Design review of the part built by this model. Coordinates are the model's own, in mm. Coordinates: 2 decimals unless noted, no trailing zeros. Order: outer loops, then holes, each group sorted by start corner. A loop starts at its lowest first (then second) coordinate and runs counter-clockwise, first axis right, second up. Notation, with made-up numbers: M 38.5,-2.75 L 77.5,-2.75 A19 cw 77.5,9.25 Z; hole C 0.25,-33.5 d11. An arc over 180 degrees is marked long. Answer in a Markdown table with one row per item.
from build123d import *

# Parameters (mm, degrees)
SKETCH1_R           = 3.05
SKETCH1_R_2         = 1.27
BOSS_EXTRUDE1_DEPTH = 5
FILLET1_R           = 3
SKETCH2_R           = 1.3
CUT_EXTRUDE1_DEPTH  = 339.464178311


with BuildPart() as part:
    # Sketch1 → Boss-Extrude1 (new body)
    with BuildSketch(Plane.XY):
        with BuildLine():
            Line((0, 0), (0, 135))
            Line((0, 135), (30, 135))
            ThreePointArc((30, 135), (32.828427125, 136.171572875), (34, 139))
            Line((34, 139), (34, 158))
            ThreePointArc((34, 158), (32.828427125, 160.828427125), (30, 162))
            Line((30, 162), (30, 193))
            Line((30, 193), (57.43, 193))
            Line((57.43, 193), (278, -29.57))
            Line((278, -29.57), (278, -57))
            Line((278, -57), (30, -57))
            Line((30, -57), (30, 0))
            Line((30, 0), (0, 0))
        make_face()
        with Locations((15, 115)):
            Circle(SKETCH1_R, mode=Mode.SUBTRACT)
        with Locations((15, 20)):
            Circle(SKETCH1_R, mode=Mode.SUBTRACT)
        with Locations((80, 148.915753479)):
            Circle(SKETCH1_R, mode=Mode.SUBTRACT)
        with Locations((228, -0.426224125)):
            Circle(SKETCH1_R, mode=Mode.SUBTRACT)
        with Locations((56.935507079, 25)):
            Circle(SKETCH1_R_2, mode=Mode.SUBTRACT)
        with Locations((102.655507079, 25)):
            Circle(SKETCH1_R_2, mode=Mode.SUBTRACT)
        with Locations((102.655507079, 5.95)):
            Circle(SKETCH1_R_2, mode=Mode.SUBTRACT)
        with Locations((56.935507079, 5.95)):
            Circle(SKETCH1_R_2, mode=Mode.SUBTRACT)
    extrude(amount=BOSS_EXTRUDE1_DEPTH)

    # Fillet1
    fillet1_edges = [part.edges().sort_by_distance(p)[0] for p in [
        (30, 162, 2.5),
        (30, 193, 2.5),
        (57.43, 193, 2.5),
        (278, -29.57, 2.5),
        (278, -57, 2.5),
        (30, -57, 2.5),
        (0, 0, 2.5),
        (0, 135, 2.5),
    ]]
    fillet(fillet1_edges, radius=FILLET1_R)

    # Sketch2 → Cut-Extrude1 (cut, through all)
    with BuildSketch(Plane.XY.offset(5)):
        with Locations((112.655507079, -30.7)):
            Circle(SKETCH2_R)
        with Locations((164.155507079, -30.7)):
            Circle(SKETCH2_R)
        with Locations((128.155507079, 25)):
            Circle(SKETCH2_R)
        with Locations((160.155507079, 25)):
            Circle(SKETCH2_R)
    extrude(amount=-CUT_EXTRUDE1_DEPTH, mode=Mode.SUBTRACT)


solid = part.part
(1) Insertion check: pin 1 Ø2.5 at (y, z) = (-23.5, 2) entering from -X; pin 2 Ø1.5 at (y, z) = (147.5, 3) entering from -X; pin 3 Ø1.5 at (x, z) = (11, 2) entering from +Y. Each pin has a flat end and moves straight along its axis. Give the tip position at first contact, or say it passes through.
Return value:
| item | result |
|---|---|
| pin 1 | stops at x = 30 |
| pin 2 | stops at x = 34 |
| pin 3 | stops at y = 135 |
(2) Add section A-A, the plane x = 228. Give the boundary of the cut face in (y, z), and give its area (3 significant figures).
Return value:
| item | result |
|---|---|
| outline | M -57,0 L -3.48,0 L -3.48,5 L -57,5 Z; M 2.62,0 L 20.88,0 L 20.88,5 L 2.62,5 Z |
| area | 359 mm2 |
(3) Add section C-C, the plane y = 115. Give the boundary of the cut face in (x, z).
Return value:
| item | result |
|---|---|
| outline | M 0,0 L 11.95,0 L 11.95,5 L 0,5 Z; M 18.05,0 L 134.73,0 L 134.73,5 L 18.05,5 Z |
(4) For line 1 along Y through (x, z) = (15, 3.9); line 2 along Y through (x, z) = (80, 2.15); line 3 along Y through (x, z) = (78, 0.9), list the stretches that pass through material, from the lowest coordinate up. Write a range as from..to.
Return value:
| item | result |
|---|---|
| line 1 | y = 0..16.95, 23.05..111.95, 118.05..135 |
| line 2 | y = -57..145.87, 151.97..170.23 |
| line 3 | y = -57..146.61, 151.22..172.24 |
(5) Add section B-B, the plane z = 3.35. Give the number of separate pieces and of enclosed holes in the cut face, and give its area (3 significant figures).
Return value:
| item | result |
|---|---|
| separate pieces | 1 |
| enclosed holes | 12 |
| area | 41,200 mm2 |
(6) Draft analysis for pull direction Y (two halves, no side actions). For faces 1 (the flat face through (166.189, 83.255, 2.465)), 2 (the flat face through (110, 42, 5)), 3 (the cylindrical face through (77.752, 150.977, 2.465)), state which applies: pulls with the +Y half, pulls with the -Y half, needs draft (parallel to the pull), parting line crosses it, or undercut.
Return value:
| item | result |
|---|---|
| face 1 | pulls with the +Y half |
| face 2 | needs draft |
| face 3 | undercut |
(7) Add section D-D, the plane x = 153.5. Give the boundary of the cut face in (y, z), and give its area (3 significant figures).
Return value:
| item | result |
|---|---|
| outline | M -57,0 L 96.06,0 L 96.06,5 L -57,5 Z |
| area | 765 mm2 |
